Input: dimensioned drawing with shaded views. Units: mm. Origin: part minimum x, y, z. A direction names the side the tool comes from. Round coordinates to 2 decimals unless told otherwise and drop trailing zeros. Loops run counter-clockwise (first coordinate to the right, second up) from the corner with the lowest first, then second, coordinate; pieces in that order, holes last.
Item 1: Section query B-B on x = 38.1. Return loops of the section in (y, z), then the cut area to 3 significant figures.
Item 2: First-contact query: P1, Ø1.3, axis at y = 44, z = 11.5, coming from the +X side; P2, Ø10, axis at x = 37.5, y = 42, coming from the +Z side. Flat tips, straight axial feed; report the tip coordinate or a pass-through.
Item 3: Section query D-D on y = 10. Return loops of the section in (x, z) (3 decimals), then the cut area to 3 significant figures.
Item 4: Pull-direction query (X, two-part tool) for the marked faces 4, 5 and 6; classes: released by +X, released by -X, zero draft, split by the parting line, or undercut.
Item 5: Section query A-A on y = 25.4. Return loops of the section in (x, z) (1 decimal).
Item 6: Ray query, L1, parallel to Y at x = 38.1, z = 7.25; L2, parallel to X at y = 25.4, z = 3; L3, parallel to X at y = 16.5, z = 11. Return the intervals inside material, ascending.
Item 7: Section query C-C on z = 6.35. Return loops of the section in (x, y), then the cut area to 3 significant figures.
Item 8: Access query for the marked faces 1, 2 and 3. Directions: +Z, -Z, +X, -X, +Y, -Y. A direction counts if a zero-diameter tool reaches every point of the face in a straight line with its end or side. Return the directions, or none.
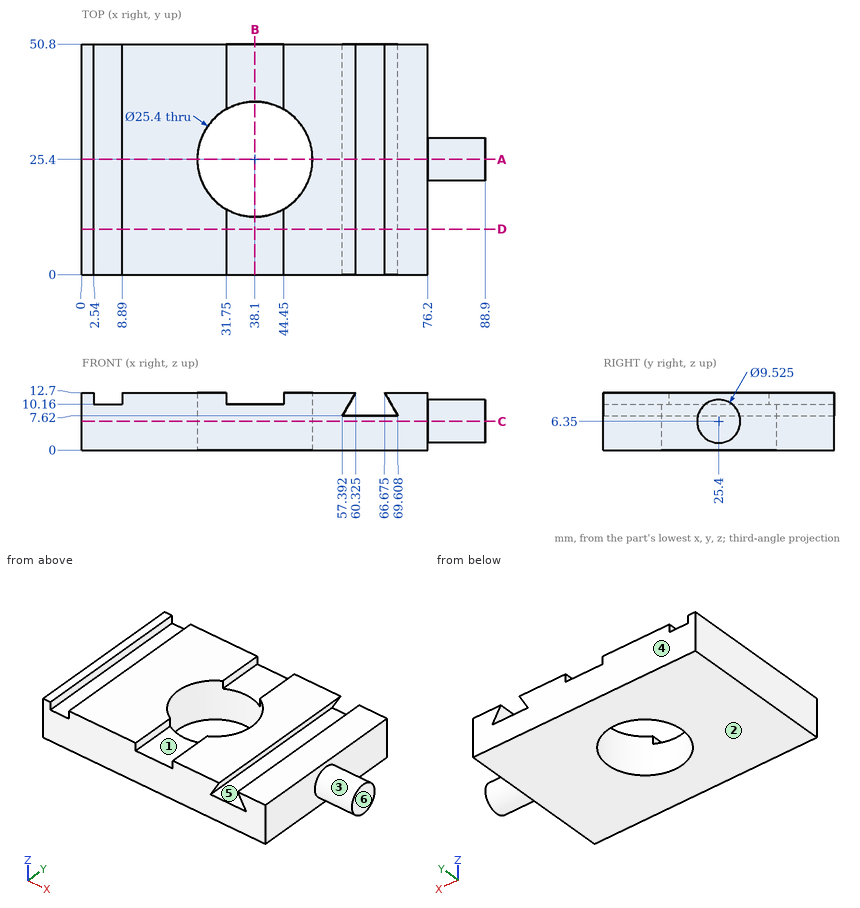
Data:
1. outline: (0, 0) - (12.7, 0) - (12.7, 10.16) - (0, 10.16) - close; (38.1, 0) - (50.8, 0) - (50.8, 10.16) - (38.1, 10.16) - close
1. area: 258 mm2
2. P1: stops at x = 76.2
2. P2: stops at z = 10.16
3. outline: (0, 0) - (76.2, 0) - (76.2, 12.7) - (66.675, 12.7) - (69.608, 7.62) - (57.392, 7.62) - (60.325, 12.7) - (44.45, 12.7) - (44.45, 10.16) - (31.75, 10.16) - (31.75, 12.7) - (8.89, 12.7) - (8.89, 10.16) - (2.54, 10.16) - (2.54, 12.7) - (0, 12.7) - close
3. area: 872 mm2
4. face 4: zero draft
4. face 5: undercut
4. face 6: released by +X
5. outline: (0, 0) - (25.4, 0) - (25.4, 12.7) - (8.9, 12.7) - (8.9, 10.2) - (2.5, 10.2) - (2.5, 12.7) - (0, 12.7) - close; (50.8, 0) - (76.2, 0) - (76.2, 1.6) - (88.9, 1.6) - (88.9, 11.1) - (76.2, 11.1) - (76.2, 12.7) - (66.7, 12.7) - (69.6, 7.6) - (57.4, 7.6) - (60.3, 12.7) - (50.8, 12.7) - close
6. L1: y = 0 to 12.7, 38.1 to 50.8
6. L2: x = 0 to 25.4, 50.8 to 88.9
6. L3: x = 0 to 2.54, 8.89 to 29.04, 47.16 to 59.34, 67.66 to 76.2
7. outline: (0, 0) - (76.2, 0) - (76.2, 20.64) - (88.9, 20.64) - (88.9, 30.16) - (76.2, 30.16) - (76.2, 50.8) - (0, 50.8) - close; hole circle Ø25.4 at (38.1, 25.4)
7. area: 3,490 mm2
8. face 1: +Z, +Y, -Y
8. face 2: -Z, +X, -X, +Y, -Y
8. face 3: +X
